Study the drawing (mm; zero at the part's minimum x, y, z) and answer. A direction names the side the tool comes from. Round coordinates to 2 decimals unless told otherwise and drop trailing zeros. Order: outer loops, then holes, each group sorted by start corner. A loop starts at its lowest first (then second) coordinate and runs counter-clockwise, first axis right, second up. Notation, with made-up numbers: (15.25, -3) - (66.25, -3) arc R7 cw to (66.25, 7) - close; hole circle Ø4 at (-27.5, -20). An arc over 180 degrees is marked (long way). Use one line per item in the form item = value. Start each with the question number.
Q1. Given P1, Ø11, axis at x = 14, z = 11.5, coming from the -Y side; P2, Ø3, axis at x = 12, y = 10, coming from the -Z side; P3, Ø5.5, axis at y = 8, z = 24, coming from the -X side, each flat-ended and moving along its own axis, determine where each tip first touches the part or whether it passes through.
Q2. Find the intervals of material crossed by line 1 (Z direction, x = 2, y = 23.55); line 2 (Z direction, x = 11, y = 22.5); line 3 (X direction, y = 23, z = 7.5), in increasing order. Write a range as [from, to].
Q3. The part is cut by section D-D on z = 7.5. Determine the outline of the cut face in (x, y).
Q4. The part is cut by section A-A on z = 2. Determine the outline of the cut face in (x, y).
Q5. The part is cut by section C-C on x = 2. Determine the outline of the cut face in (y, z).
Q6. The part is cut by section B-B on x = 11. Determine the outline of the cut face in (y, z), plus the area to 3 significant figures.
Q7. Which of the six approach directions +Z, -Z, +X, -X, +Y, -Y give full straight-line access (tool end or side, diameter ignored) to the marked faces 1, 2, 3, 4 and 5?
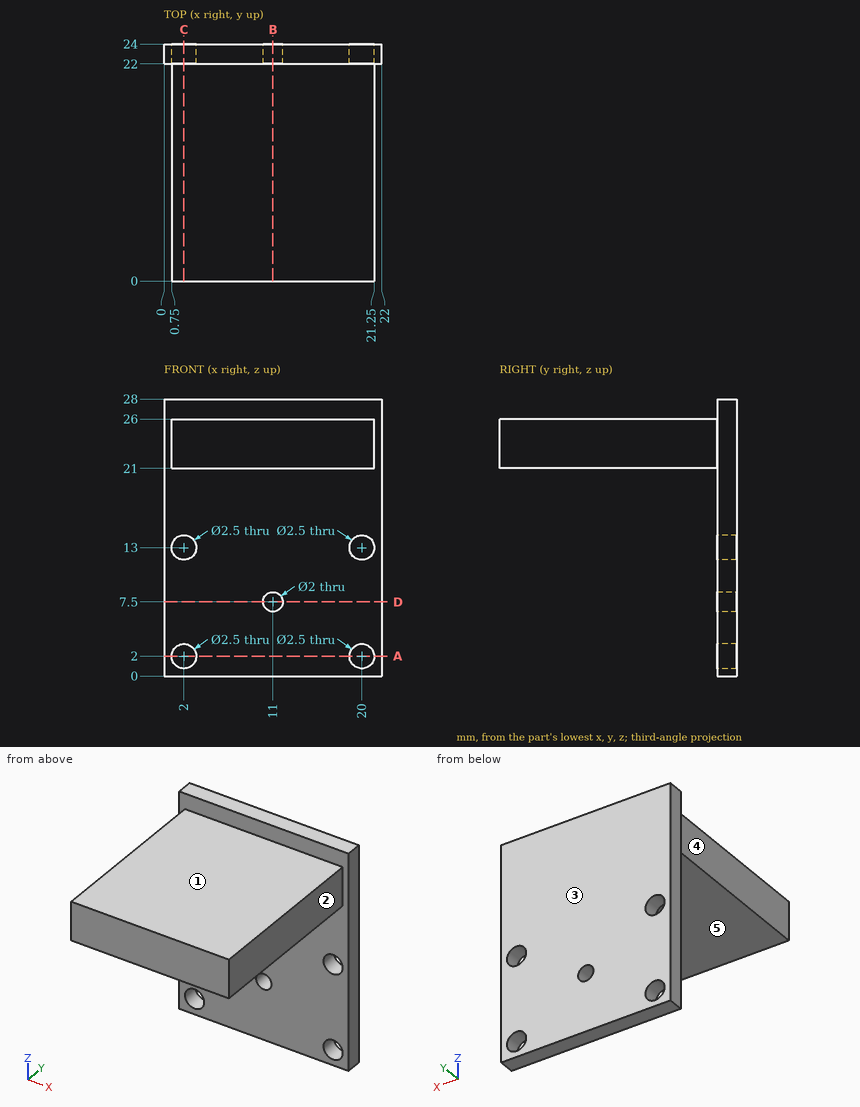
Found:
q1.P1 = 22
q1.P2 = 21
q1.P3 = 0.75
q2.line_1 = [0, 0.75], [3.25, 11.75], [14.25, 28]
q2.line_2 = [0, 6.5], [8.5, 28]
q2.line_3 = [0, 10], [12, 22]
q3.outline = (0, 22) - (10, 22) - (10, 24) - (0, 24) - close; (12, 22) - (22, 22) - (22, 24) - (12, 24) - close
q4.outline = (0, 22) - (0.75, 22) - (0.75, 24) - (0, 24) - close; (3.25, 22) - (18.75, 22) - (18.75, 24) - (3.25, 24) - close; (21.25, 22) - (22, 22) - (22, 24) - (21.25, 24) - close
q5.outline = (0, 21) - (22, 21) - (22, 14.25) - (24, 14.25) - (24, 28) - (22, 28) - (22, 26) - (0, 26) - close; (22, 0) - (24, 0) - (24, 0.75) - (22, 0.75) - close; (22, 3.25) - (24, 3.25) - (24, 11.75) - (22, 11.75) - close
q6.outline = (0, 21) - (22, 21) - (22, 8.5) - (24, 8.5) - (24, 28) - (22, 28) - (22, 26) - (0, 26) - close; (22, 0) - (24, 0) - (24, 6.5) - (22, 6.5) - close
q6.area = 162 mm²
q7.face_1 = +Z, +X, -X, -Y
q7.face_2 = +Z, -Z, +X, -Y
q7.face_3 = +Z, -Z, +X, -X, +Y
q7.face_4 = +Z, -Z, -X, -Y
q7.face_5 = -Z, +X, -X, -Y
